Geometry check sheet. Reference: the model listing, model coordinates, mm. A direction names the side the tool comes from. Round coordinates to 2 decimals unless told otherwise and drop trailing zeros. Loops run counter-clockwise (first coordinate to the right, second up) from the corner with the lowest first, then second, coordinate; pieces in that order, holes last.
```python
from build123d import *

# Parameters (mm, degrees)
BOSS_EXTRUDE1_DEPTH   = 57.15
M4_CLEARANCE_HOLE1_D  = 4.5
SKETCH7_R             = 22.225
CUT_EXTRUDE1_DEPTH    = 28.575
F_8_CLEARANCE_HOLE1_D = 4.4958


with BuildPart() as part:
    # Sketch1 → Boss-Extrude1 (new body)
    with BuildSketch(Plane(origin=(0, 0, 0), x_dir=(0, 0, -1), z_dir=(1, 0, 0))):
        with BuildLine():
            Line((3.175, -19.05), (3.175, 28.575))
            ThreePointArc((3.175, 28.575), (2.24506403, 30.82006403), (0, 31.75))
            Line((0, 31.75), (-3.175, 31.75))
            Line((-3.175, 31.75), (-3.175, -31.75))
            Line((-3.175, -31.75), (60.325, -31.75))
            Line((60.325, -31.75), (60.325, -28.575))
            ThreePointArc((60.325, -28.575), (59.39506403, -26.32993597), (57.15, -25.4))
            Line((57.15, -25.4), (9.525, -25.4))
            ThreePointArc((9.525, -25.4), (5.034871939, -23.540128061), (3.175, -19.05))
        make_face()
    extrude(amount=BOSS_EXTRUDE1_DEPTH)

    # M4 Clearance Hole1 (through all)
    with Locations(Plane(origin=(0, -31.75, 0), x_dir=(-1, 0, 0), z_dir=(0, -1, 0))):
        with Locations((-45.575, 50.8), (-11.575, 50.8), (-11.575, 16.7894), (-45.575, 16.7894)):
            Hole(M4_CLEARANCE_HOLE1_D / 2)

    # Sketch7 → Cut-Extrude1 (cut, symmetric)
    with BuildSketch(Plane(origin=(0, 0, -3.175), x_dir=(-1, 0, 0), z_dir=(0, 0, -1))):
        with Locations(Location((-28.575, -2.3114, 0), (0, 0, 311.136639748))):  # turned: the seam where the file's is
            Circle(SKETCH7_R)
    extrude(amount=CUT_EXTRUDE1_DEPTH, both=True, mode=Mode.SUBTRACT)

    # #8 Clearance Hole1 (through all)
    with Locations(Plane(origin=(0, 0, -3.175), x_dir=(-1, 0, 0), z_dir=(0, 0, -1))):
        with Locations((-50.8, 19.9136), (-6.35, 19.9136)):
            Hole(F_8_CLEARANCE_HOLE1_D / 2)


solid = part.part
```
1) Mould release check, pull along X, two halves, no side actions. Record for faces 3 (the face through (9.79, -28.53, -49.43)), 4 (the face through (28, 31.75, 2)), 5 (the face through (0, -12, -3)): +X half, -X half, draft (parallel to the pull), parting line (faces both ways), or undercut.
Report:
face 3: undercut
face 4: draft
face 5: -X half
2) Sectioned sample at B-B, the plane y = 12. Record the cut outline in (x, z) (3 decimals).
Report:
outline: (0, -3.175) - (11.571, -3.175) - (11.571, 3.175) - (0, 3.175) - close; (45.579, -3.175) - (57.15, -3.175) - (57.15, 3.175) - (45.579, 3.175) - close
3) Access from +Z, -Z, +X, -X, +Y, -Y to the whole of each face (thin tool, end or side, straight path). Record for faces 1 (the face through (28, -25.4, -34)), 2 (the face through (28, -30, -60.325)).
Report:
face 1: -Z, +X, -X, +Y
face 2: -Z, +X, -X, +Y, -Y
4) Sectioned sample at C-C, the plane x = 46.5. Record the cut outline in (y, z) (3 decimals).
Report:
outline: (-31.75, -60.325) - (-28.575, -60.325) arc R3.175 ccw to (-25.4, -57.15) - (-25.4, -52.851) - (-31.75, -52.851) - close; (-31.75, -48.749) - (-25.4, -48.749) - (-25.4, -18.84) - (-31.75, -18.84) - close; (-31.75, -14.738) - (-25.4, -14.738) - (-25.4, -9.525) arc R6.35 cw to (-19.05, -3.175) - (-15.451, -3.175) - (-15.451, 3.175) - (-31.75, 3.175) - close; (10.828, -3.175) - (28.575, -3.175) arc R3.175 ccw to (31.75, 0) - (31.75, 3.175) - (10.828, 3.175) - close
5) Sectioned sample at D-D, the plane x = 21. Record the cut outline in (y, z) (3 decimals).
Report:
outline: (-31.75, -60.325) - (-28.575, -60.325) arc R3.175 ccw to (-25.4, -57.15) - (-25.4, -9.525) arc R6.35 cw to (-23.206, -4.724) - (-23.206, 3.175) - (-31.75, 3.175) - close; (18.583, -3.175) - (28.575, -3.175) arc R3.175 ccw to (31.75, 0) - (31.75, 3.175) - (18.583, 3.175) - close
6) Scan lines: line 1 along X through (y, z) = (20.5, -3); line 2 along Y through (x, z) = (51, -27.5); line 3 along Z through (x, y) = (5, -7) (3 decimals). Record each from-to range of solid material in increasing order.
Report:
line 1: x = 0 to 4.18, 8.52 to 48.63, 52.97 to 57.15
line 2: y = -31.75 to -25.4
line 3: z = -3.175 to 3.175
7) Sectioned sample at A-A, the plane z = -50.8. Record the cut outline in (x, y) (3 decimals), then the cut area to 3 significant figures.
Report:
outline: (0, -31.75) - (9.325, -31.75) - (9.325, -25.4) - (0, -25.4) - close; (13.825, -31.75) - (43.325, -31.75) - (43.325, -25.4) - (13.825, -25.4) - close; (47.825, -31.75) - (57.15, -31.75) - (57.15, -25.4) - (47.825, -25.4) - close
area: 306 mm2
8) Gauge pin test, flat ends, axial feed: pin 1 (1.5 mm diameter, centred on x = 32, z = -6, fed in from +Y); pin 2 (5 mm diameter, centred on x = 11.575, z = -50.8, fed in from +Y); pin 3 (6 mm diameter, centred on x = 50.8, y = 19.91, fed in from -Z) (3 decimals); pin 4 (4 mm diameter, centred on x = 10, z = -51.5, fed in from -Y). Record the tip position at first contact, or that the pin passes through.
Report:
pin 1: stops at y = -24.15
pin 2: stops at y = -25.4
pin 3: stops at z = -3.175
pin 4: stops at y = -31.75
